Input: part model. Units: mm. Frame: model coordinates. Face numbers are marked on the shaded views. A direction names the side the tool comes from. Give positions to 0.01 mm unless a question says otherwise; leave off trailing zeros. Order: outer loops, then holes, each group sorted by start corner. A loop starts at its lowest first (then second) coordinate and runs counter-clockwise, first axis right, second up. Notation, with made-up numbers: (51, 11.25) - (58, 11.25) arc R16 cw to (58, 33.25) - close; hole circle Ø1 at (27.5, 68). An arc over 180 degrees is marked (long way). Answer in a Markdown table with one row per item. Add a question column.
1. Contact query for flat-ended pins moving along their axis: pin 1 (8.5 mm diameter, centred on y = 82, z = -3.5, fed in from +X); pin 2 (3 mm diameter, centred on x = -38, y = 2, fed in from -Z); pin 3 (14 mm diameter, centred on y = -161, z = 0, fed in from +X); pin 4 (11 mm diameter, centred on y = -161, z = 0, fed in from +X). Output: stop coordinate, or through.
2. Mould query, pull axis X, two halves, no side actions, for the marked faces 4, 5 and 6. Classes: released by +X, released by -X, zero draft, split by the parting line, or undercut.
3. Ray query, line 1 (Y direction, x = -22.05, z = 0); line 2 (X direction, y = -139, z = 10); line 3 (Y direction, x = 23.5, z = 29.5). Return the intervals inside material, ascending. Write a range as [from, to].
4. Section query A-A on y = -161. Return loops of the section in (x, z).
5. Access query for the marked faces 1, 2 and 3. Directions: +Z, -Z, +X, -X, +Y, -Y. A direction counts if a zero-diameter tool reaches every point of the face in a straight line with its end or side. Return the directions, or none.
6. Section query C-C on y = 9.5. Return loops of the section in (x, z).
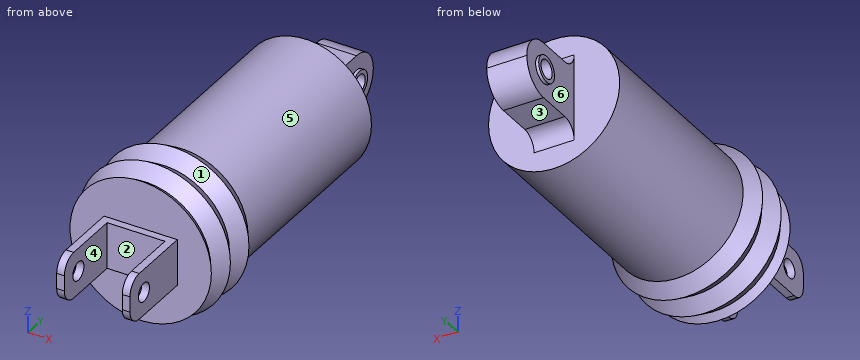
```python
from build123d import *

# Parameters (mm, degrees)
SZKIC2_W                    = 26
SZKIC2_H                    = 36
DODANIE_WYCI_GNI_CIE1_DEPTH = 51
SZKIC3_W                    = 47.5
SZKIC3_H                    = 30
DODANIE_WYCI_GNI_CIE2_DEPTH = 5
SZKIC4_W                    = 5
SZKIC4_H                    = 30
DODANIE_WYCI_GNI_CIE3_DEPTH = 46
SZKIC5_R                    = 6
WYTNIJ_WYCI_GNI_CIE1_DEPTH  = 197.7283515
SZKIC6_R                    = 6
WYTNIJ_WYCI_GNI_CIE2_DEPTH  = 46
DODANIE_WYCI_GNI_CIE4_START = 2
SZKIC8_R                    = 8.5
SZKIC8_R_2                  = 6
DODANIE_WYCI_GNI_CIE4_DEPTH = 2
ZAOKR_GLENIE1_R             = 18
ZAOKR_GLENIE2_R             = 10
ZAOKR_GLENIE3_R             = 10


with BuildPart() as part:
    # Szkic1 → Obrót1 (revolve)
    with BuildSketch(Plane.XY, mode=Mode.PRIVATE) as obr_t1_sk:
        Polygon((-42.5, 0), (-42.5, 53), (0, 53), (0, -125), (-45.81662479, -125), (-42.5, -120), (-49.133249581, -110), (-42.5, -100), (-49.133249581, -90), (-42.5, -80), align=None)
    revolve(obr_t1_sk.sketch.rotate(Axis((0, -125, 0), (0, 1, 0)), 180), axis=Axis((0, -125, 0), (0, 1, 0)))

    # Szkic2 → Dodanie-wyciągnięcie1 (add)
    with BuildSketch(Plane(origin=(0, 53, 0), x_dir=(1, 0, 0), z_dir=(0, 1, 0))):
        Rectangle(SZKIC2_W, SZKIC2_H)
    extrude(amount=DODANIE_WYCI_GNI_CIE1_DEPTH)

    # Szkic3 → Dodanie-wyciągnięcie2 (add)
    with BuildSketch(Plane.XZ.offset(125)):
        Rectangle(SZKIC3_W, SZKIC3_H)
    extrude(amount=DODANIE_WYCI_GNI_CIE2_DEPTH)

    # Szkic4 → Dodanie-wyciągnięcie3 (add)
    with BuildSketch(Plane.XZ.offset(130)):
        with Locations((-21.25, 0)):
            Rectangle(SZKIC4_W, SZKIC4_H)
        with Locations((21.25, 0)):
            Rectangle(SZKIC4_W, SZKIC4_H)
    extrude(amount=DODANIE_WYCI_GNI_CIE3_DEPTH)

    # Szkic5 → Wytnij-wyciągnięcie1 (cut, through all)
    with BuildSketch(Plane(origin=(23.75, 0, 0), x_dir=(0, 0, -1), z_dir=(1, 0, 0))):
        with Locations((0, -161)):
            Circle(SZKIC5_R)
    extrude(amount=-WYTNIJ_WYCI_GNI_CIE1_DEPTH, mode=Mode.SUBTRACT)

    # Szkic6 → Wytnij-wyciągnięcie2 (cut)
    with BuildSketch(Plane(origin=(13, 0, 0), x_dir=(0, 0, -1), z_dir=(1, 0, 0))):
        with Locations((0, 86)):
            Circle(SZKIC6_R)
    extrude(amount=-WYTNIJ_WYCI_GNI_CIE2_DEPTH, mode=Mode.SUBTRACT)

    # Szkic8 → Dodanie-wyciągnięcie4 (add)
    with BuildSketch(Plane(origin=(13, 0, 0), x_dir=(0, 0, -1), z_dir=(1, 0, 0)).offset(DODANIE_WYCI_GNI_CIE4_START)):
        with Locations(Location((0, 86, 0), (0, 0, 180))):
            Circle(SZKIC8_R)
        with Locations((0, 86)):
            Circle(SZKIC8_R_2, mode=Mode.SUBTRACT)
    dodanie_wyci_gni_cie4 = extrude(amount=-DODANIE_WYCI_GNI_CIE4_DEPTH)

    # Lustro1: Dodanie-wyciągnięcie4 across plane
    add(dodanie_wyci_gni_cie4.mirror(Plane(origin=(0, 0, 0), x_dir=(0, 0, 1), z_dir=(1, 0, 0))))

    # Zaokrąglenie1
    zaokr_glenie1_edges = [part.edges().sort_by_distance(p)[0] for p in [
        (0, 104, 18),
        (0, 104, -18),
    ]]
    fillet(zaokr_glenie1_edges, radius=ZAOKR_GLENIE1_R - 0.0001)  # a hair under: the kernel refuses the full size

    # Zaokrąglenie2
    zaokr_glenie2_edges = [part.edges().sort_by_distance(p)[0] for p in [
        (0, 53, -18),
        (0, 53, 18),
    ]]
    fillet(zaokr_glenie2_edges, radius=ZAOKR_GLENIE2_R)

    # Zaokrąglenie3
    zaokr_glenie3_edges = [part.edges().sort_by_distance(p)[0] for p in [
        (-21.25, -176, -15),
        (-21.25, -176, 15),
        (21.25, -176, 15),
        (21.25, -176, -15),
    ]]
    fillet(zaokr_glenie3_edges, radius=ZAOKR_GLENIE3_R)


solid = part.part
```
Answer:
| question | item | result |
|---|---|---|
| 1 | pin 1 | stops at x = 15 |
| 1 | pin 2 | stops at z = -21.77 |
| 1 | pin 3 | stops at x = 23.75 |
| 1 | pin 4 | passes through |
| 2 | face 4 | undercut |
| 2 | face 5 | split by the parting line |
| 2 | face 6 | released by -X |
| 3 | line 1 | y = [-176, -167], [-155, 53] |
| 3 | line 2 | x = [-23.75, -18.75], [18.75, 23.75] |
| 3 | line 3 | y = [-125, 53] |
| 4 | outline | (-23.75, -15) - (-18.75, -15) - (-18.75, -6) - (-23.75, -6) - close; (-23.75, 6) - (-18.75, 6) - (-18.75, 15) - (-23.75, 15) - close; (18.75, -15) - (23.75, -15) - (23.75, -6) - (18.75, -6) - close; (18.75, 6) - (23.75, 6) - (23.75, 15) - (18.75, 15) - close |
| 5 | face 1 | none |
| 5 | face 2 | +Z, -Z, -Y |
| 5 | face 3 | -Z, +X, -X, +Y |
| 6 | outline | circle Ø85 at (0, 0) |
